Autodesk Inventor part; units mm, degrees
ref_plane "YZ Plane" through (0, 0, 0) normal (1, 0, 0) x (0, 1, 0)
ref_plane "XZ Plane" through (0, 0, 0) normal (0, 1, 0) x (-1, 0, 0)
ref_plane "XY Plane" through (0, 0, 0) normal (0, 0, 1) x (1, 0, 0)
sketch "Skizze1" plane through (0, 0, 0) normal (0, 1, 0) x (-1, 0, 0)
  arc A0 (-2.1739, -19.8815) -> (-2.1739, 19.8815) centre (0, 0) ccw
  arc A1 (-47.6304, 14.9111) -> (-47.6304, -14.9111) centre (-46, 0) ccw
  line L0 (-2.1739, 19.8815) -> (-47.6304, 14.9111)
  line L1 (-2.1739, -19.8815) -> (-47.6304, -14.9111)
  line L2 (45.0235, 0) -> (-115.148, 0) construction
  arc A2 (-1.8478, -16.8993) -> (-1.8478, 16.8993) centre (0, 0) ccw
  arc A3 (-47.3043, 11.9289) -> (-47.3043, -11.9289) centre (-46, 0) ccw
  line L3 (-1.8478, 16.8993) -> (-47.3043, 11.9289)
  line L4 (-1.8478, -16.8993) -> (-47.3043, -11.9289)
  dimension "d0" = 40
  dimension "d1" = 30
  dimension "d2" = 46
  dimension "d3" = 3
  dimension "d4" = 3
extrude "Extrusion1" add sketch "Skizze1" along normal blind 1
properties part number "Dichtungsgummi"
Geometry check sheet. Reference: the model listing, model coordinates, mm. A direction names the side the tool comes from. Give positions to 0.01 mm unless a question says otherwise; leave off trailing zeros. Write each loop counter-clockwise with the first axis right and the second up, starting at its lowest first coordinate (ties: lowest second). Pieces come first, ordered by that corner, then holes.
1) Section check B-B, the plane z = 0. Record the boundary of the cut face in (x, y).
2) Material ranges on L1, parallel to Z at x = 0, y = 0.45; L2, parallel to X at y = 0.8, z = -7 (3 decimals); L3, parallel to Z at x = -9, y = 0.8, recorded low to high.
3) Access from +Z, -Z, +X, -X, +Y, -Y to the whole of each face (thin tool, end or side, straight path). Record for faces 4 (the cylindrical face through (60.997, 0.493, -0.307)), 5 (the cylindrical face through (58, 0.5, -0.2)).
4) Section check C-C, the plane y = 0.4. Record the boundary of the cut face in (x, z), and give its area (3 significant figures).
5) Release check for a two-part mould opening along X. For faces 1 (the cylindrical face through (-16.995, 0.493, 0.4)), 2 (the flat face through (21, 0, 15)), 3 (the flat face through (24.58, 0.49, -17.43)) record: pulls with the +X half, pulls with the -X half, needs draft (parallel to the pull), parting line crosses it, or undercut.
6) Section check A-A, the plane x = 0. Record the boundary of the cut face in (y, z).
Computed:
1. outline: (-20, 0) - (-17, 0) - (-17, 1) - (-20, 1) - close; (58, 0) - (61, 0) - (61, 1) - (58, 1) - close
2. L1: z = -20 to -17, 17 to 20
2. L2: x = -18.735 to -15.492, 55.747 to 59.266
2. L3: z = -17.86 to -14.42, 14.42 to 17.86
3. face 4: +X, +Y, -Y
3. face 5: +Y, -Y
4. outline: (2.17, -19.88) - (47.63, -14.91) arc R15 ccw to (47.63, 14.91) - (2.17, 19.88) arc R20 ccw (long way) to start; hole (1.85, -16.9) - (47.3, -11.93) arc R12 ccw to (47.3, 11.93) - (1.85, 16.9) arc R17 ccw (long way) to start
4. area: 579 mm2
5. face 1: undercut
5. face 2: needs draft
5. face 3: pulls with the +X half
6. outline: (0, -20) - (1, -20) - (1, -17) - (0, -17) - close; (0, 17) - (1, 17) - (1, 20) - (0, 20) - close
